from build123d import *

# Parameters (mm, degrees)
SKETCH1_W               = 16
SKETCH1_H               = 39.5
BOSS_EXTRUDE1_DEPTH     = 15
SKETCH2_W               = 10
SKETCH2_H               = 33.5
CUT_EXTRUDE1_DEPTH      = 3
CUT_EXTRUDE2_DEPTH      = 45.274710615
CUT_EXTRUDE2_DEPTH_BACK = 45.274710615
SKETCH3_R               = 1.6
CUT_EXTRUDE3_DEPTH      = 3
CUT_EXTRUDE3_DEPTH_BACK = 46.180194776
SKETCH4_R               = 1.6
SKETCH5_R               = 2.5
CUT_EXTRUDE4_DEPTH      = 20
SKETCH8_R               = 4.25
CUT_EXTRUDE5_DEPTH      = 4
SKETCH9_W               = 23.074046619
SKETCH9_H               = 49.619494536
CUT_EXTRUDE6_DEPTH      = 5


with BuildPart() as part:
    # Sketch1 → Boss-Extrude1 (new body)
    with BuildSketch(Plane(origin=(0, 0, 0), x_dir=(1, 0, 0), z_dir=(0, 1, 0))):
        with Locations((8, 19.75)):
            Rectangle(SKETCH1_W, SKETCH1_H)
    extrude(amount=BOSS_EXTRUDE1_DEPTH)

    # Sketch2 → Cut-Extrude1 (cut)
    with BuildSketch(Plane(origin=(0, 15, 0), x_dir=(1, 0, 0), z_dir=(0, 1, 0))):
        with Locations((8, 19.75)):
            Rectangle(SKETCH2_W, SKETCH2_H)
    extrude(amount=-CUT_EXTRUDE1_DEPTH, mode=Mode.SUBTRACT)

    # Sketch3 → Cut-Extrude2 (cut, two sides: drawn at the far end of the back side and taken through both)
    with BuildSketch(Plane(origin=(0, 12, 0), x_dir=(1, 0, 0), z_dir=(0, 1, 0)).offset(-CUT_EXTRUDE2_DEPTH_BACK)):
        with Locations(Location((2.7, 2.5, 0), (0, 0, 270))):
            Circle(SKETCH3_R)
    extrude(amount=CUT_EXTRUDE2_DEPTH + CUT_EXTRUDE2_DEPTH_BACK, mode=Mode.SUBTRACT)

    # Sketch4 → Cut-Extrude3 (cut, two sides: drawn at the far end of the back side and taken through both)
    with BuildSketch(Plane(origin=(0, 15, 0), x_dir=(1, 0, 0), z_dir=(0, 1, 0)).offset(-CUT_EXTRUDE3_DEPTH_BACK)):
        with Locations(Location((13.3, 2.5, 0), (0, 0, 100.806922875))):
            Circle(SKETCH4_R)
        with Locations(Location((2.7, 17, 0), (0, 0, 79.193077125))):
            Circle(SKETCH4_R)
        with Locations(Location((2.5, 36, 0), (0, 0, 18.209956864))):
            Circle(SKETCH4_R)
    extrude(amount=CUT_EXTRUDE3_DEPTH + CUT_EXTRUDE3_DEPTH_BACK, mode=Mode.SUBTRACT)

    # Sketch5 → Cut-Extrude4 (cut)
    with BuildSketch(Plane(origin=(0, 12, 0), x_dir=(1, 0, 0), z_dir=(0, 1, 0))):
        with Locations(Location((8, 26, 0), (0, 0, 270))):
            Circle(SKETCH5_R)
    extrude(amount=-CUT_EXTRUDE4_DEPTH, mode=Mode.SUBTRACT)

    # Sketch8 → Cut-Extrude5 (cut)
    with BuildSketch(Plane(origin=(0, 12, 0), x_dir=(1, 0, 0), z_dir=(0, 1, 0))):
        with Locations(Location((8, 26, 0), (0, 0, 270))):
            Circle(SKETCH8_R)
    extrude(amount=-CUT_EXTRUDE5_DEPTH, mode=Mode.SUBTRACT)

    # Sketch9 → Cut-Extrude6 (cut)
    with BuildSketch(Plane.XZ):
        with Locations((7.55036405, -17.360616358)):
            Rectangle(SKETCH9_W, SKETCH9_H)
    extrude(amount=-CUT_EXTRUDE6_DEPTH, mode=Mode.SUBTRACT)


solid = part.part
Check sheet for the modelled part. Datum: model origin and axes. Units: mm. A direction names the side the tool comes from. Give positions to 0.01 mm unless a question says otherwise; leave off trailing zeros. Loops run counter-clockwise (first coordinate to the right, second up) from the corner with the lowest first, then second, coordinate; pieces in that order, holes last. Notation, with made-up numbers: M -33.5,45.25 L 11.5,45.25 A25 cw 11.5,61.25 Z; hole C 19,-22.75 d11. An arc over 180 degrees is marked long. Answer as a JSON object with one key per item and string values. Group by question number.
Q1. Cross-section at D-D on z = -2.5. Record the cut outline in (x, y), then the cut area to 3 significant figures.
Q2. Cross-section at C-C on y = 13.25. Record the cut outline in (x, z), then the cut area to 3 significant figures.
Q3. Access from +Z, -Z, +X, -X, +Y, -Y to the whole of each face (thin tool, end or side, straight path). Record for faces 1 (the flat face through (13, 14, -20)), 2 (the flat face through (0, 10, -19)).
Q4. Cross-section at B-B on y = 6.25. Record the cut outline in (x, z), then the cut area to 3 significant figures.
Q5. Go/stop test with flat-tipped pins: P1, Ø4.5, axis at x = 8, z = -26, coming from the -Y side; P2, Ø5, axis at x = 7.5, z = -20.5, coming from the +Y side. Record where each tip stops, or that it passes through.
Q6. Cross-section at A-A on z = -28. Record the cut outline in (x, y).
Q7. Release check for a two-part mould opening along Z. For faces 3 (the flat face through (8, 14, -36.5)), 4 (the flat face through (8, 10, 0)), 5 (the flat face through (13.2, 15, -20)), 6 (the cylindrical face through (2.09, 9.93, -1.02)) record: released by +Z, released by -Z, zero draft, split by the parting line, or undercut.
Q8. Material ranges on line 1 along X through (y, z) = (8.5, -2.5); line 2 along X through (y, z) = (14.25, -24); line 3 along Z through (x, y) = (13.3, 9.25), recorded low to high. Write a range as [from, to].
Evaluation:
{
 "1": {"outline": "M 0,5 L 1.1,5 L 1.1,15 L 0,15 Z; M 4.3,5 L 11.7,5 L 11.7,15 L 4.3,15 Z; M 14.9,5 L 16,5 L 16,15 L 14.9,15 Z", "area": "96.0 mm2"},
 "2": {"outline": "M 0,-39.5 L 16,-39.5 L 16,0 L 0,0 Z; hole M 3,-34.48 A1.6 ccw long 4.02,-36.5 L 13,-36.5 L 13,-4.07 A1.6 ccw long 11.78,-3 L 4.22,-3 A1.6 ccw long 3,-4.07 L 3,-15.43 A1.6 ccw long 3,-18.57 Z", "area": "271 mm2"},
 "3": {"face 1": "+Y", "face 2": "+Z, -Z, -X, +Y, -Y"},
 "4": {"outline": "M 0,-39.5 L 16,-39.5 L 16,0 L 0,0 Z; hole C 2.5,-36 d3.2; hole C 2.7,-17 d3.2; hole C 2.7,-2.5 d3.2; hole C 8,-26 d5; hole C 13.3,-2.5 d3.2", "area": "580 mm2"},
 "5": {"P1": "passes through", "P2": "stops at y = 12"},
 "6": {"outline": "M 0,5 L 6.5,5 L 6.5,8 L 4.25,8 L 4.25,12 L 3,12 L 3,15 L 0,15 Z; M 9.5,5 L 16,5 L 16,15 L 13,15 L 13,12 L 11.75,12 L 11.75,8 L 9.5,8 Z"},
 "7": {"face 3": "undercut", "face 4": "released by +Z", "face 5": "zero draft", "face 6": "undercut"},
 "8": {"line 1": "x = [0, 1.1], [4.3, 11.7], [14.9, 16]", "line 2": "x = [0, 3], [13, 16]", "line 3": "z = [-39.5, -4.1], [-0.9, 0]"}
}
